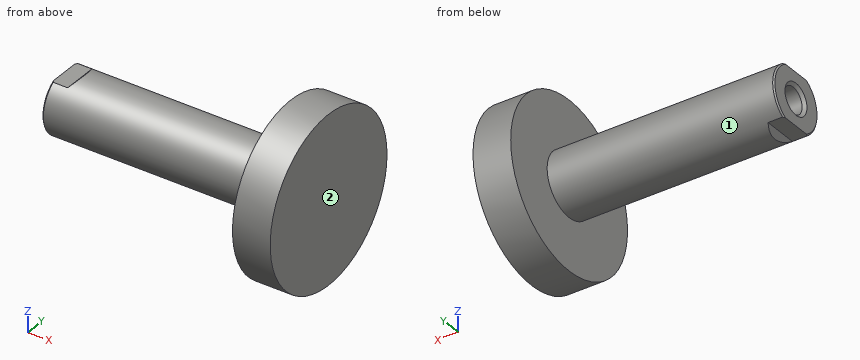
Autodesk Inventor part; units mm, degrees
ref_plane "for_body_XY" through (0, 0, 0) normal (1, 0, 0) x (0, 0, -1)
ref_plane "for_body_YZ" through (0, 0, 0) normal (0, 0, -1) x (0, 1, 0)
ref_plane "for_body_ZX" through (0, 0, 0) normal (0, 1, 0) x (1, 0, 0)
sketch "Sketch_12" plane through (0, 0, 0) normal (0, 0, 1) x (1, 0, 0)
  line L0 (0, 0) -> (-7, 0)
  line L1 (-7, 0) -> (-7, 5.75)
  line L2 (-7, 5.75) -> (-6.75, 6)
  line L3 (-6.75, 6) -> (0, 6)
  line L4 (0, 6) -> (0, 0)
  line L5 (0, 0) -> (-7, 0)
revolve "Revolution1" add sketch "Sketch_12" angle 360 about axis through (0, 0, 0) along (1, 0, 0)
sketch "Sketch_16" plane through (0, 0, 0) normal (0, 0, 1) x (1, 0, 0)
  line L0 (43.5, 0) -> (0, 0)
  line L1 (0, 0) -> (0, 6)
  line L2 (0, 6) -> (36.3, 6)
  line L3 (36.3, 6) -> (36.3, 15.95)
  line L4 (36.3, 15.95) -> (43.5, 15.95)
  line L5 (43.5, 15.95) -> (43.5, 0)
  line L6 (43.5, 0) -> (0, 0)
revolve "Revolution2" add sketch "Sketch_16" angle 360 about axis through (43.5, 0, 0) along (1, 0, 0)
sketch "Sketch_13" plane through (0, 0, 0) normal (0, 1, 0) x (-1, 0, 0)
  line L0 (17, -10) -> (17, 10)
  line L1 (17, 10) -> (-1, 10)
  line L2 (-1, 10) -> (4, 5)
  line L3 (4, 5) -> (7, 5)
  line L4 (7, 5) -> (7, -5)
  line L5 (7, -5) -> (4, -5)
  line L6 (4, -5) -> (-1, -10)
  line L7 (-1, -10) -> (17, -10)
extrude "Extrusion1" cut sketch "Sketch_13" along normal mid plane 20
sketch "Sketch4" plane through (-7, -2.8395, 5) normal (-1, 0, 0) x (0, 0, 1)
  point P0 (-5, 2.8395)
hole "Hole1" at (-7, 0, 0) direction (1, 0, 0) diameter 4.917 depth 14.4 tip angle 120 countersink diameter 6 countersink angle 90
ref_plane "for_body_XY" through (0, 0, 0) normal (1, 0, 0) x (0, 0, -1)
ref_plane "for_body_YZ" through (0, 0, 0) normal (0, 0, -1) x (0, 1, 0)
ref_plane "for_body_ZX" through (0, 0, 0) normal (0, 1, 0) x (1, 0, 0)
ref_plane "for_nut_XY" through (-17.5, 0, 0) normal (-1, 0, 0) x (0, 0, -1)
ref_plane "for_nut_YZ" through (-17.5, 0, 0) normal (0, 0, -1) x (0, -1, 0)
ref_plane "for_nut_ZX" through (-17.5, 0, 0) normal (0, -1, 0) x (-1, 0, 0)
properties part number "SDA-32x2525_r"
Could you check a few things on this model? Use its own coordinates, in mm. Face numbers are marked on the shaded views. A direction names the side the tool comes from. Round coordinates to 2 decimals unless told otherwise and drop trailing zeros. Order: outer loops, then holes, each group sorted by start corner. A loop starts at its lowest first (then second) coordinate and runs counter-clockwise, first axis right, second up. Notation, with made-up numbers: M -1.75,35 L 54.25,35 A13 cw 54.25,59 Z; hole C 42,53 d11. An arc over 180 degrees is marked long. One line per question, with ' | ' between items. Start each with the question number.
(1) Please list where these lines run through material, in increasing order: line 1 along Z through (x, y) = (-0.25, 0); line 2 along Z through (x, y) = (-3.25, 0); line 3 along X through (y, z) = (-13.5, -1.5).
(2) For the marked faces 1 and 2, which set-ups out of +Z, -Z, +X, -X, +Y, -Y let a thin tool reach every point of the face, with its end or its side?
(3) Suppose I cut it at A-A on x = 2.5. List the corners of the cut face in (y, z) for me.
(4) Suppose I cut it at B-B on x = 13. List the corners of the cut face in (y, z) for me, then the cut area to 3 significant figures.
(5) For P1, Ø10, axis at y = -8, z = -6, coming from the -X side; P2, Ø8, axis at x = 36, y = 8, coming from the +Z side; P3, Ø2.5, axis at x = -6, y = 0, coming from the +Z side; P4, Ø8, axis at x = 30.5, z = -8.5, coming from the +Y side, each with a flat end and sliding along its axis, tell me the tip position at first contact or that it passes through.
Geometry results:
1) line 1: -6 to -2.46, 2.46 to 6 | line 2: -5.75 to -2.46, 2.46 to 5.75 | line 3: 36.3 to 43.5
2) face 1: -X | face 2: +Z, -Z, +X, +Y, -Y
3) outline: C 0,0 d12; hole C 0,0 d4.92
4) outline: C 0,0 d12 | area: 113 mm²
5) P1: x = -7 | P2: z = 15.44 | P3: z = 5 | P4: y = 3.97
